Autodesk Inventor part; units mm, degrees
ref_plane "YZ Plane" through (0, 0, 0) normal (1, 0, 0) x (0, 1, 0)
ref_plane "XZ Plane" through (0, 0, 0) normal (0, 1, 0) x (-1, 0, 0)
ref_plane "XY Plane" through (0, 0, 0) normal (0, 0, 1) x (1, 0, 0)
sketch "Sketch1" plane through (0, 0, 0) normal (0, 1, 0) x (-1, 0, 0)
  line L0 (0, 0) -> (31.5, 0)
  line L1 (223, -6) -> (246, -6)
  line L2 (246, -6) -> (246, 6)
  line L3 (246, 6) -> (223, 6)
  line L4 (223, 6) -> (223, -6)
  line L5 (223, -6) -> (246, 6) construction
  line L6 (246, -6) -> (223, 6) construction
  line L7 (234.5, 0) -> (249, 0) construction
  line L8 (234.5, 0) -> (220, 0) construction
  line L9 (0, 0) -> (18.5, 0) construction
  line L10 (223, 0) -> (240, 0) construction
  line L11 (0, 0) -> (-10.5, 0)
  line L12 (-20, 0) -> (-20, 20)
  line L13 (-20, 20) -> (253, 20)
  line L14 (253, 20) -> (253, 0)
  line L15 (253, 0) -> (240, 0) construction
  line L16 (253, 0) -> (246, 0)
  line L17 (-10.5, 10.5) -> (31.5, 10.5)
  line L18 (31.5, 10.5) -> (31.5, -10.5)
  line L19 (31.5, -10.5) -> (-10.5, -10.5)
  line L20 (-10.5, -10.5) -> (-10.5, 10.5)
  line L21 (-10.5, 10.5) -> (31.5, -10.5) construction
  line L22 (31.5, 10.5) -> (-10.5, -10.5) construction
  line L23 (-14.5, 5) -> (35.5, 5) construction
  line L24 (35.5, 5) -> (35.5, -5) construction
  line L25 (35.5, -5) -> (-14.5, -5) construction
  line L26 (-14.5, -5) -> (-14.5, 5) construction
  line L27 (-14.5, 5) -> (35.5, -5) construction
  line L28 (35.5, 5) -> (-14.5, -5) construction
  line L29 (31.5, 0) -> (223, 0)
  line L30 (-10.5, 0) -> (-20, 0)
  line L31 (-20, 0) -> (0, 0) construction
  point P0 (10.5, 0)
  point P1 (10.5, 0)
  dimension "d21" = 240
  dimension "d22" = 23
  dimension "d23" = 12
  dimension "d24" = 6
  dimension "d25" = 14.5
  dimension "d26" = 14.5
  dimension "d28" = 18.5
  dimension "d37" = 20
  dimension "d38" = 20
  dimension "d39" = 42
  dimension "d40" = 21
  dimension "d41" = 50
  dimension "d42" = 10
  dimension "d43" = 10.5
  dimension "d52" = 7
extrude "Extrusion1" add sketch "Sketch1" along normal blind 3.5 contours L18 L17 L20 L30 L12 L13 L14 L16 L2 L3 L4 L29
hole "Hole3" at (0, 0, 0) at (-249, 0, 0) at (-220, 0, 0) at (14.5, 0, 5) at (-35.5, 0, 5) direction (0, 1, 0) diameter 2 end through all
fillet "Fillet1" [suppressed]
mirror "Mirror1" about plane through (-31.5, 0, 0) normal (0, 0, -1)
properties part number "segment2a" material "Plywood, Finish"
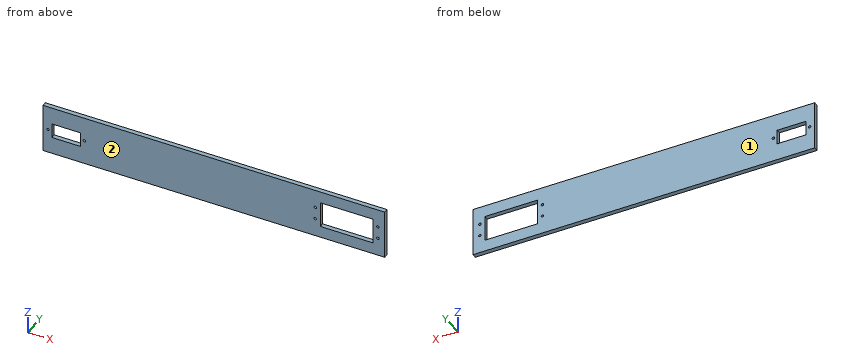
Source: CAD feature listing. Evaluate the final solid. Frame: model axes, mm. Face numbers are marked on the shaded views. Round coordinates to 2 decimals unless told otherwise and drop trailing zeros. Loops run counter-clockwise (first coordinate to the right, second up) from the corner with the lowest first, then second, coordinate; pieces in that order, holes last. Notation, with made-up numbers: M 64.5,43.25 L 80.5,43.25 A16 ccw 80.5,61.25 Z; hole C 65,27.25 d1. An arc over 180 degrees is marked long. Return JSON: item names as keys, results as strings. Group by question number.
1. Mould query, pull axis Y, two halves, no side actions, for the marked faces 1 and 2. Classes: released by +Y, released by -Y, zero draft, split by the parting line, or undercut.
2. Pin query (flat end, axial travel): pin 1 (1.8 mm diameter, centred on x = -220, z = 0, fed in from -Y). Return the tip coordinate at first contact, or that it passes through.
3. Section query A-A on y = 1.7. State how many separate pieces and enclosed holes the cut face has, and give its area (3 significant figures).
4. Material intervals for line 1 along Z through (x, y) = (-35.5, 1.55); line 2 along X through (y, z) = (0.85, -5); line 3 along X through (y, z) = (1.4, 3), sorted ascending. Write a range as from..to.
5. Section query B-B on x = -22. Output: boundary loops of the cut face in (y, z).
Checks:
{
 "1": {"face 1": "released by +Y", "face 2": "released by -Y"},
 "2": {"pin 1": "passes through"},
 "3": {"separate pieces": "1", "enclosed holes": "8", "area": "9,740 mm²"},
 "4": {"line 1": "z = -20..-6, -4..4, 6..20", "line 2": "x = -253..-246, -223..-36.5, -34.5..-31.5, 10.5..13.5, 15.5..20", "line 3": "x = -253..-246, -223..-31.5, 10.5..20"},
 "5": {"outline": "M 0,-20 L 3.5,-20 L 3.5,-10.5 L 0,-10.5 Z; M 0,10.5 L 3.5,10.5 L 3.5,20 L 0,20 Z"}
}
